For this review, take the finished solid that the model builds, in its own axes (mm). Round coordinates to 2 decimals unless told otherwise and drop trailing zeros. Write each loop counter-clockwise with the first axis right and the second up, starting at its lowest first coordinate (ties: lowest second). Pieces come first, ordered by that corner, then holes. Notation, with made-up numbers: (55.25, 21.25) -> (111.25, 21.25) arc R5 cw to (111.25, 25.25) -> close; hole circle Ø4 at (58, -8). An arc over 180 degrees is marked (long way). Answer in a Markdown table with one row per item.
from build123d import *

# Parameters (mm, degrees)
SKETCH_1_W          = 140
SKETCH_1_H          = 50
EXTRUDE_1_DEPTH     = 3
SKETCH_2_W          = 20
SKETCH_2_H          = 20
CUT_EXTRUDE_1_DEPTH = 3
SKETCH_3_W          = 60
SKETCH_3_H          = 30
CUT_EXTRUDE_2_DEPTH = 3
SKETCH_4_R          = 2
CUT_EXTRUDE_4_DEPTH = 3
SKETCH_5_R          = 2
CUT_EXTRUDE_5_DEPTH = 3
FILLET_1_R          = 2


with BuildPart() as part:
    # 草图1 → 凸台-拉伸1 (new body)
    with BuildSketch(Plane.XY):
        Rectangle(SKETCH_1_W, SKETCH_1_H)
    extrude(amount=EXTRUDE_1_DEPTH)

    # 草图2 → 切除-拉伸1 (cut)
    with BuildSketch(Plane.XY.offset(3)):
        with Locations((-50, -5)):
            Rectangle(SKETCH_2_W, SKETCH_2_H)
        with Locations((50, -5)):
            Rectangle(SKETCH_2_W, SKETCH_2_H)
    extrude(amount=-CUT_EXTRUDE_1_DEPTH, mode=Mode.SUBTRACT)

    # 草图3 → 切除-拉伸2 (cut)
    with BuildSketch(Plane.XY.offset(3)):
        with Locations((0, -10)):
            Rectangle(SKETCH_3_W, SKETCH_3_H)
    extrude(amount=-CUT_EXTRUDE_2_DEPTH, mode=Mode.SUBTRACT)

    # 草图4 → 切除-拉伸4 (cut)
    with BuildSketch(Plane.XY.offset(3)):
        with Locations((-65, -20)):
            Circle(SKETCH_4_R)
        with Locations((-35, -20)):
            Circle(SKETCH_4_R)
        with Locations(Location((65, -20, 0), (0, 0, 180))):
            Circle(SKETCH_4_R)
        with Locations(Location((35, -20, 0), (0, 0, 180))):
            Circle(SKETCH_4_R)
    extrude(amount=-CUT_EXTRUDE_4_DEPTH, mode=Mode.SUBTRACT)

    # 草图5 → 切除-拉伸5 (cut)
    with BuildSketch(Plane.XY.offset(3)):
        with Locations((-65, 15)):
            Circle(SKETCH_5_R)
        with Locations((-35, 15)):
            Circle(SKETCH_5_R)
        with Locations(Location((35, 15, 0), (0, 0, 180))):
            Circle(SKETCH_5_R)
        with Locations(Location((65, 15, 0), (0, 0, 180))):
            Circle(SKETCH_5_R)
    extrude(amount=-CUT_EXTRUDE_5_DEPTH, mode=Mode.SUBTRACT)

    # 圆角1
    fillet_1_edges = [part.edges().sort_by_distance(p)[0] for p in [
        (30, 5, 1.5),
        (30, -25, 1.5),
        (-30, -25, 1.5),
        (-30, 5, 1.5),
        (70, -25, 1.5),
        (-70, -25, 1.5),
        (-70, 25, 1.5),
        (70, 25, 1.5),
    ]]
    fillet(fillet_1_edges, radius=FILLET_1_R)


solid = part.part
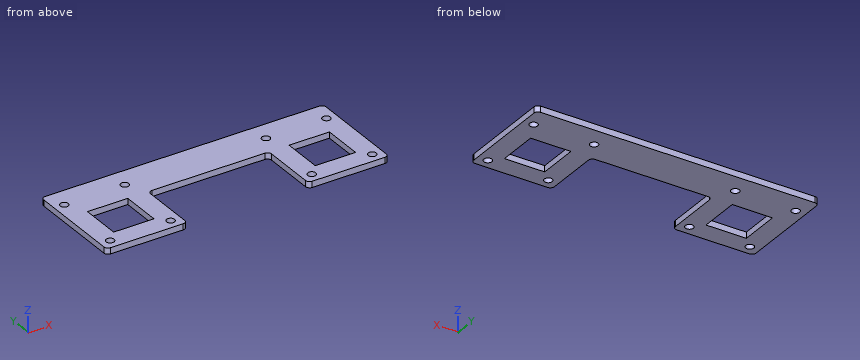
1) Consider section B-B on y = -20. State the section outline as (x, z) points.
Solved:
| item | result |
|---|---|
| outline | (-70, 0) -> (-67, 0) -> (-67, 3) -> (-70, 3) -> close; (-63, 0) -> (-37, 0) -> (-37, 3) -> (-63, 3) -> close; (-33, 0) -> (-30, 0) -> (-30, 3) -> (-33, 3) -> close; (30, 0) -> (33, 0) -> (33, 3) -> (30, 3) -> close; (37, 0) -> (63, 0) -> (63, 3) -> (37, 3) -> close; (67, 0) -> (70, 0) -> (70, 3) -> (67, 3) -> close |
2) Consider section A-A on x = 65. State the section outline as (y, z) points.
Solved:
| item | result |
|---|---|
| outline | (-25, 0) -> (-22, 0) -> (-22, 3) -> (-25, 3) -> close; (-18, 0) -> (13, 0) -> (13, 3) -> (-18, 3) -> close; (17, 0) -> (25, 0) -> (25, 3) -> (17, 3) -> close |
3) Consider section D-D on z = 1.15. State how many separate pieces and enclosed holes the cut face has, then the cut area to 3 significant figures.
Solved:
| item | result |
|---|---|
| separate pieces | 1 |
| enclosed holes | 10 |
| area | 4,300 mm² |
4) For line 1 (Y direction, x = -35, z = 1.65); line 2 (Y direction, x = -56, z = 0.2); line 3 (X direction, y = 2, z = 0.3), list the stretches that pass through material, from the lowest coordinate up. Write a range as [from, to].
Solved:
| item | result |
|---|---|
| line 1 | [-25, -22], [-18, 13], [17, 25] |
| line 2 | [-25, -15], [5, 25] |
| line 3 | [-70, -60], [-40, -30], [30, 40], [60, 70] |
5) Clearance check with a flat-ended pin moving along its axis: pin 1 Ø12 at (x, y) = (-13, -6) entering from -Z. State where the tip first meets the part, or that it passes through.
Solved:
| item | result |
|---|---|
| pin 1 | through |
6) Consider section C-C on x = 43. State the section outline as (y, z) points.
Solved:
| item | result |
|---|---|
| outline | (-25, 0) -> (-15, 0) -> (-15, 3) -> (-25, 3) -> close; (5, 0) -> (25, 0) -> (25, 3) -> (5, 3) -> close |
